```python
from build123d import *

# Parameters (mm, degrees)
BOSS_EXTRUDE1_DEPTH = 6
SKETCH3_R           = 0.25
CUT_EXTRUDE1_DEPTH  = 16.575086945


with BuildPart() as part:
    # Sketch1 → Boss-Extrude1 (new, symmetric)
    with BuildSketch(Plane(origin=(0, 0, 0), x_dir=(1, 0, 0), z_dir=(0, 1, 0))):
        Polygon((0, 7.505553499), (-6.5, 3.75277675), (-6.5, -3.75277675), (0, -7.505553499), (6.5, -3.75277675), (6.5, 3.75277675), align=None)
    extrude(amount=BOSS_EXTRUDE1_DEPTH, both=True)

    # Sketch2 → Cut-Revolve3 (revolve, cut)
    with BuildSketch(Plane.ZY):
        Polygon((-0.75, 6), (-7.505553499, 0.33141755), (-7.505553499, 6), align=None)
    revolve(axis=Axis((0, 0, 0), (0, 1, 0)), mode=Mode.SUBTRACT)

    # Sketch3 → Cut-Extrude1 (cut, through all)
    with BuildSketch(Plane(origin=(0, 6, 0), x_dir=(1, 0, 0), z_dir=(0, 1, 0))):
        with Locations(Location((0, 0, 0), (0, 0, 270))):
            Circle(SKETCH3_R)
    extrude(amount=-CUT_EXTRUDE1_DEPTH, mode=Mode.SUBTRACT)

    # Sketch4 → Cut-Revolve4 (revolve, cut)
    with BuildSketch(Plane(origin=(0, 0, 0), x_dir=(0, 0, -1), z_dir=(1, 0, 0))):
        Polygon((0, -6), (-5, -6), (-5, 0), (-1.8375, 0), (-1.5875, 0.25), (-1.5875, 3.232815039), (0, 5.5), align=None)
    revolve(axis=Axis((0, 6, 0), (0, -1, 0)), mode=Mode.SUBTRACT)


solid = part.part
```
For this review, take the finished solid that the model builds, in its own axes (mm). A direction names the side the tool comes from. Coordinates: 2 decimals unless noted, no trailing zeros. Write each loop counter-clockwise with the first axis right and the second up, starting at its lowest first coordinate (ties: lowest second). Pieces come first, ordered by that corner, then holes.
(1) Add section C-C on y = 2.25. Give the boundary of the cut face in (x, z) (1 decimal), then the cut area to 3 significant figures.
(2) Tool access review of faces 1 (the face through (-6.5, -2, 0)), 2 (the face through (1.55, 1.76, -0.34)): name each direction out of +Z, -Z, +X, -X, +Y, -Y from which nothing blocks a thin tool from reaching the whole face with its end or side.
(3) Add section A-A on y = -4.25. Give the boundary of the cut face in (x, z).
(4) Add section B-B on z = 0. Give the boundary of the cut face in (x, y).
(5) For pin 1 Ø4 at (x, z) = (-2, 4) entering from -Y; pin 2 Ø2 at (x, z) = (3, -0.5) entering from -Y; pin 3 Ø4 at (x, y) = (3, 1) entering from -Z; pin 4 Ø6 at (x, y) = (-4, 3.5) entering from -Z, all flat-tipped, find the tip position at first contact; note any pin that passes through.
(6) The part is to be moulded in two halves that separate along Z. For faces 3 (the face through (0.598, 4.626, -0.133)), 4 (the face through (1.9, 5, 0.4)), 5 (the face through (6.5, -2, 0)), say which applies: +Z half, -Z half, draft (parallel to the pull), parting line (faces both ways), or undercut.
(7) Add section D-D on y = 4.5. Give the boundary of the cut face in (x, z), then the cut area to 3 significant figures.
(8) Wall thickness on probe 1 along X at (y, z) = (-2.8, 0); probe 2 along X at (y, z) = (2.45, 0); probe 3 along Z at (x, y) = (0.5, 1.75): over which ranges is each line inside the solid? List them lowest first.
Answer sheet:
1. outline: circle Ø10.4 at (0, 0); hole circle Ø3.2 at (0, 0)
1. area: 77.7 mm2
2. face 1: +Z, -Z, -X, +Y, -Y
2. face 2: -Y
3. outline: (-6.5, -3.75) - (0, -7.51) - (6.5, -3.75) - (6.5, 3.75) - (0, 7.51) - (-6.5, 3.75) - close; hole circle Ø10 at (0, 0)
4. outline: (-6.5, -6) - (-5, -6) - (-5, 0) - (-1.84, 0) - (-1.59, 0.25) - (-1.59, 3.23) - (-0.25, 5.14) - (-0.25, 6) - (-0.75, 6) - (-6.5, 1.18) - close; (0.25, 5.14) - (1.59, 3.23) - (1.59, 0.25) - (1.84, 0) - (5, 0) - (5, -6) - (6.5, -6) - (6.5, 1.18) - (0.75, 6) - (0.25, 6) - close
5. pin 1: stops at y = -6
5. pin 2: stops at y = 0
5. pin 3: stops at z = -6.92
5. pin 4: stops at z = -6.22
6. face 3: undercut
6. face 4: parting line
6. face 5: draft
7. outline: circle Ø5.08 at (0, 0); hole circle Ø1.4 at (0, 0)
7. area: 18.7 mm2
8. probe 1: x = -6.5 to -5, 5 to 6.5
8. probe 2: x = -4.98 to -1.59, 1.59 to 4.98
8. probe 3: z = -5.79 to -1.51, 1.51 to 5.79
